Part model, mm, in its own coordinate system. Face numbers are marked on the shaded views. A direction names the side the tool comes from. Give positions to 0.01 mm unless a question says otherwise; leave off trailing zeros. Order: outer loops, then holes, each group sorted by start corner. A loop starts at its lowest first (then second) coordinate and runs counter-clockwise, first axis right, second up. Notation, with made-up numbers: (3.25, 11.25) - (16.25, 11.25) arc R5 ccw to (16.25, 17.25) - close; hole circle Ø8 at (15, 9.25). An arc over 180 degrees is marked (long way). Use a Markdown table: item, result. Add a question column.
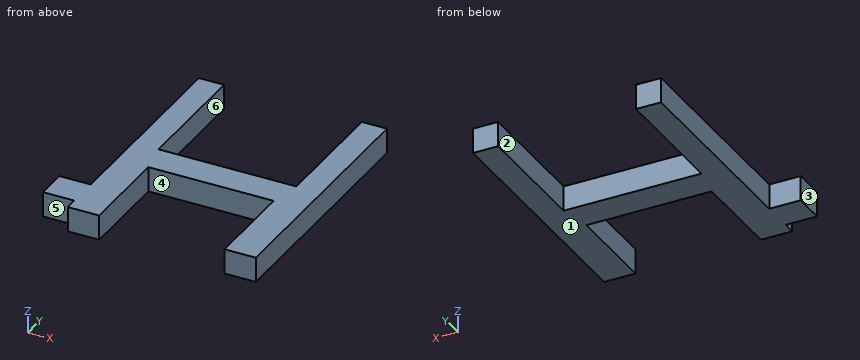
from build123d import *

# Parameters (mm, degrees)
P_IDAT_VYSUNUT_M1_DEPTH  = 4
SKICA2_W                 = 20
SKICA2_H                 = 4
P_IDAT_VYSUNUT_M2_DEPTH  = 15
SKICA3_W                 = 5.5
SKICA3_H                 = 3
ODEBRAT_VYSUNUT_M1_DEPTH = 15
SKICA4_W                 = 20
SKICA4_H                 = 15
ODEBRAT_VYSUNUT_M2_DEPTH = 15
SKICA5_W                 = 4
SKICA5_H                 = 4
P_IDAT_VYSUNUT_M3_DEPTH  = 20


with BuildPart() as part:
    # Skica1 → Přidat vysunutím1 (new body)
    with BuildSketch(Plane.XY):
        Polygon((0, 0), (5, 0), (5, -2), (10, -2), (10, 4.082474227), (10, 13), (30, 13), (30, -2), (35, -2), (35, 18), (5, 18), (5, 5), (0, 5), align=None)
    extrude(amount=P_IDAT_VYSUNUT_M1_DEPTH)

    # Skica2 → Přidat vysunutím2 (add)
    with BuildSketch(Plane(origin=(0, 18, 0), x_dir=(1, 0, 0), z_dir=(0, 1, 0))):
        with Locations((20, -2)):
            Rectangle(SKICA2_W, SKICA2_H)
    extrude(amount=P_IDAT_VYSUNUT_M2_DEPTH)

    # Skica3 → Odebrat vysunutím1 (cut)
    with BuildSketch(Plane.XY.offset(4)):
        with Locations((20, 28)):
            Rectangle(SKICA3_W, SKICA3_H)
    extrude(amount=-ODEBRAT_VYSUNUT_M1_DEPTH, mode=Mode.SUBTRACT)

    # Skica4 → Odebrat vysunutím2 (cut)
    with BuildSketch(Plane.XY.offset(4)):
        with Locations((20, 25.5)):
            Rectangle(SKICA4_W, SKICA4_H)
    extrude(amount=-ODEBRAT_VYSUNUT_M2_DEPTH, mode=Mode.SUBTRACT)

    # Skica5 → Přidat vysunutím3 (add)
    with BuildSketch(Plane(origin=(0, 18, 0), x_dir=(1, 0, 0), z_dir=(0, 1, 0))):
        with Locations((7, -2)):
            Rectangle(SKICA5_W, SKICA5_H)
        with Locations((33, -2)):
            Rectangle(SKICA5_W, SKICA5_H)
    extrude(amount=P_IDAT_VYSUNUT_M3_DEPTH)


solid = part.part
1. Cut at A-A (y = 4.5). Write the cut outline in (x, z).
2. Tool access for the marked faces 4, 5 and 6: list every direction of +Z, -Z, +X, -X, +Y, -Y with a clear straight run to the whole face (end or side of a thin tool).
3. Cut at B-B (z = 0.85). Write the cut outline in (x, y).
4. Mould opens along X. For the marked faces 1, 2 and 3 say: released by +X, released by -X, zero draft, split by the parting line, or undercut.
5. Cut at C-C (y = 27). Write the cut outline in (x, z), plus the area to 3 significant figures.
6. Drill centre lines: probe 1 along X at (y, z) = (7, 1); probe 2 along X at (y, z) = (31.5, 1.25); probe 3 along Y at (x, z) = (14, 3.65). Where is each one in solid material? Low to high. Write a range as [from, to].
7. Pin check, flat tips, straight feed: P1, Ø2, axis at x = 21.5, z = 2, coming from the -Y side; P2, Ø1.2, axis at y = 28.5, z = 2.5, coming from the -X side; P3, Ø2, axis at x = 21.5, z = 2.5, coming from the +Y side; P4, Ø6, axis at x = 30, y = 19, coming from the +Z side. Stop position of each tip, or through.
8. Cut at D-D (x = 21). Write the cut outline in (y, z), plus the area to 3 significant figures.
Responses:
| question | item | result |
|---|---|---|
| 1 | outline | (0, 0) - (10, 0) - (10, 4) - (0, 4) - close; (30, 0) - (35, 0) - (35, 4) - (30, 4) - close |
| 2 | face 4 | +Z, -Z, -Y |
| 2 | face 5 | +Z, -Z, -X, -Y |
| 2 | face 6 | +Z, -Z, +Y |
| 3 | outline | (0, 0) - (5, 0) - (5, -2) - (10, -2) - (10, 13) - (30, 13) - (30, -2) - (35, -2) - (35, 38) - (31, 38) - (31, 18) - (9, 18) - (9, 38) - (5, 38) - (5, 5) - (0, 5) - close |
| 4 | face 1 | zero draft |
| 4 | face 2 | undercut |
| 4 | face 3 | released by -X |
| 5 | outline | (5, 0) - (9, 0) - (9, 4) - (5, 4) - close; (31, 0) - (35, 0) - (35, 4) - (31, 4) - close |
| 5 | area | 32.0 mm² |
| 6 | probe 1 | x = [5, 10], [30, 35] |
| 6 | probe 2 | x = [5, 9], [31, 35] |
| 6 | probe 3 | y = [13, 18] |
| 7 | P1 | stops at y = 13 |
| 7 | P2 | stops at x = 5 |
| 7 | P3 | stops at y = 18 |
| 7 | P4 | stops at z = 4 |
| 8 | outline | (13, 0) - (18, 0) - (18, 4) - (13, 4) - close |
| 8 | area | 20.0 mm² |
